```python
from build123d import *

# Parameters (mm, degrees)
F0_W     = 254
F0_H     = 177.8
F1_DEPTH = 34.925
F2_DEPTH = 88.9
F3_DEPTH = 76.2
F4_DEPTH = 25.4


with BuildPart() as f1:
    # F0 (on Front) → F1 (new body, symmetric)
    with BuildSketch(Plane.XZ):
        with Locations((736.6, -88.9)):
            Rectangle(F0_W, F0_H)
    extrude(amount=F1_DEPTH, both=True)

    # F0 (on Front) → F2 (join, symmetric)
    with BuildSketch(Plane.XZ):
        with BuildLine():
            Line((609.6, 0), (-127, 0))
            ThreePointArc((-127, 0), (-606.4601433609, 48.1137509537), (-1066.8, 190.5362860105))
            Line((-1066.8, 190.5362860105), (-1066.8, 70.8278600943))
            ThreePointArc((-1066.8, 70.8278600943), (-547.6947262881, -114.8211673081), (0, -177.8))
            Line((0, -177.8), (609.6, -177.8))
            Line((609.6, -177.8), (609.6, 0))
        make_face()
    extrude(amount=F2_DEPTH, both=True)

    # F0 (on Front) → F3 (join, symmetric)
    with BuildSketch(Plane.XZ):
        with BuildLine():
            Line((-1066.8, 70.8278600943), (-1066.8, 190.5362860105))
            ThreePointArc((-1066.8, 190.5362860105), (-1111.4504024994, 209.9506576069), (-1155.7, 230.2619694521))
            Line((-1155.7, 230.2619694521), (-1155.7, 116.963348915))
            ThreePointArc((-1155.7, 116.963348915), (-1111.4893986594, 93.4342993063), (-1066.8, 70.8278600943))
        make_face()
    extrude(amount=F3_DEPTH, both=True)

    # F0 (on Front) → F4 (cut, symmetric)
    with BuildSketch(Plane.XZ):
        with BuildLine():
            Line((-1066.8, 70.8278600943), (-1066.8, 190.5362860105))
            ThreePointArc((-1066.8, 190.5362860105), (-1111.4504024994, 209.9506576069), (-1155.7, 230.2619694521))
            Line((-1155.7, 230.2619694521), (-1155.7, 116.963348915))
            ThreePointArc((-1155.7, 116.963348915), (-1111.4893986594, 93.4342993063), (-1066.8, 70.8278600943))
        make_face()
    extrude(amount=F4_DEPTH, both=True, mode=Mode.SUBTRACT)


solid = f1.part
```
Geometry: final body of the model. Coordinates: model frame, mm. A direction names the side the tool comes from. Round coordinates to 2 decimals unless told otherwise and drop trailing zeros. Loops run counter-clockwise (first coordinate to the right, second up) from the corner with the lowest first, then second, coordinate; pieces in that order, holes last. Notation, with made-up numbers: (25.25, 24) -> (47.25, 24) arc R37 cw to (47.25, 62) -> close; hole circle Ø11 at (73, 26.5). An arc over 180 degrees is marked (long way). Use one line per item in the form item = value. Start each with the question number.
1) Section C-C on x = 727. Output: boundary loops of the cut face in (y, z) (3 decimals).
2) Access query for faces 1 (the flat face through (735, -34.925, -88)), 2 (the flat face through (-1112, 76.2, 152)), 3 (the flat face through (-1112, -25.4, 152)). Directions: +Z, -Z, +X, -X, +Y, -Y. A direction counts if a zero-diameter tool reaches every point of the face in a straight line with its end or side. Return the directions, or none.
3) First-contact query: P1, Ø8, axis at x = -558.5, y = -4, coming from the -Z side; P2, Ø1.5, axis at y = -15, z = 14.5, coming from the -X side; P3, Ø6, axis at x = -382, y = -17.5, coming from the -Z side. Flat tips, straight axial feed; report the tip coordinate or a pass-through.
4) Section A-A on z = -142. Output: boundary loops of the cut face in (x, y) (1 decimal).
5) Section B-B on y = -7.5. Output: boundary loops of the cut face in (x, z), then the cut area to 3 significant figures.
6) Section D-D on z = -67. Output: boundary loops of the cut face in (x, y) (3 decimals), then the cut area to 3 significant figures.
7) Line query: L1, parallel to Z at x = 46, y = -64; L2, parallel to Y at x = 717, z = -9.5 (3 decimals); L3, parallel to Z at x = -89, y = 67. Output: solid intervals per line, ascending.
Response:
q1.outline = (-34.925, -177.8) -> (34.925, -177.8) -> (34.925, 0) -> (-34.925, 0) -> close
q2.face_1 = +Z, -Z, +X, -Y
q2.face_2 = +Z, -Z, -X, +Y
q2.face_3 = +Z, -Z, -X
q3.P1 = -113.22
q3.P2 = -945.72
q3.P3 = -147.85
q4.outline = (-414.1, -88.9) -> (609.6, -88.9) -> (609.6, -34.9) -> (863.6, -34.9) -> (863.6, 34.9) -> (609.6, 34.9) -> (609.6, 88.9) -> (-414.1, 88.9) -> close
q5.outline = (-1066.8, 70.83) arc R2413 ccw to (0, -177.8) -> (863.6, -177.8) -> (863.6, 0) -> (-127, 0) arc R2413 cw to (-1066.8, 190.54) -> close
q5.area = 315,000 mm^2
q6.outline = (-722.803, -88.9) -> (609.6, -88.9) -> (609.6, -34.925) -> (863.6, -34.925) -> (863.6, 34.925) -> (609.6, 34.925) -> (609.6, 88.9) -> (-722.803, 88.9) -> close
q6.area = 255,000 mm^2
q7.L1 = -177.8 to 0
q7.L2 = -34.925 to 34.925
q7.L3 = -176.16 to 0
